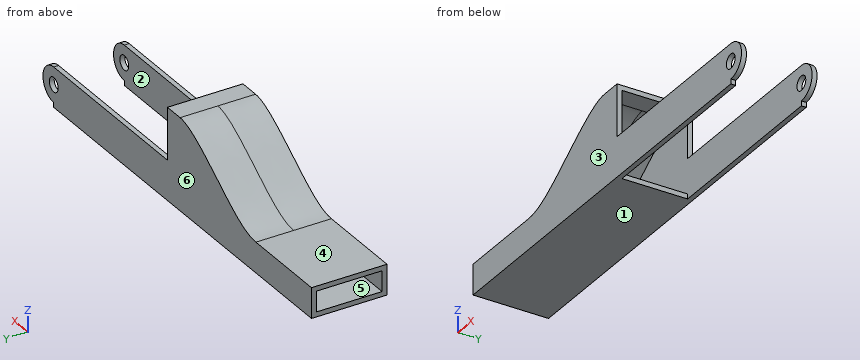
from build123d import *

# Parameters (mm, degrees)
F0_W     = 45
F0_H     = 8.5
F0_H_2   = 1.2
F0_W_2   = 22
F0_H_3   = 5
F1_DEPTH = 1.2
F2_DEPTH = 9.2
F3_D     = 3.5


# Not quite as in the source:
# - the dataset's text gives a spline's control points without its knots; the knots are read off the source's solid


with BuildPart() as f1:
    # F0 (on Front) → F1 (new body)
    with BuildSketch(Plane.XZ):
        with BuildLine():
            Line((47.5, -1.5), (47.5, -10))
            ThreePointArc((47.5, -10), (51.75, -5.75), (47.5, -1.5))
        make_face()
        with Locations((25, -5.75)):
            Rectangle(F0_W, F0_H)
        with Locations((25, -10.6)):
            Rectangle(F0_W, F0_H_2)
        with BuildLine():
            Line((-32.5, -10), (-2.5, -10))
            Line((-2.5, -10), (-2.5, 10))
            add(Edge.make_bspline(
                [(-32.5, -5), (-27.5803674012, -5), (-17.2100449751, 2.2275754238), (-6.0579581186, 10), (-2.5, 10)],
                knots=[0, 0, 0, 0, 0.5090778259, 1, 1, 1, 1], degree=3))
            Line((-32.5, -5), (-32.5, -10))
        make_face()
        Polygon((-2.5, -10), (2.5, -10), (2.5, -1.5), (2.5, 10), (-2.5, 10), align=None)
        with Locations((-43.5, -7.5)):
            Rectangle(F0_W_2, F0_H_3)
    extrude(amount=F1_DEPTH)

    # F0 (on Front) → F2 (join)
    with BuildSketch(Plane.XZ):
        with BuildLine():
            add(Edge.make_bspline(
                [(-32.5, -5), (-27.5803674012, -5), (-17.2100449751, 2.2275754238), (-6.0579581186, 10), (-2.5, 10)],
                knots=[0, 0, 0, 0, 0.5090778259, 1, 1, 1, 1], degree=3))
            Line((-2.5, 10), (2.5, 10))
            Line((2.5, 10), (2.5, 11.2))
            Line((2.5, 11.2), (-2.5, 11.2))
            add(Edge.make_bspline(
                [(-32.5, -3.8), (-31.4389363622, -3.8), (-29.2200835852, -3.4091842374), (-25.6037921172, -1.8183804645), (-21.7862624056, 0.5093473763), (-17.819156486, 3.2622809958), (-13.7265020427, 6.1236212623), (-10.3779360475, 8.2729183736), (-7.8194468713, 9.6607467479), (-5.973100675, 10.4877178879), (-4.2025331466, 11.0487112992), (-3.0621946213, 11.2), (-2.5, 11.2)],
                knots=[0, 0, 0, 0, 0.125, 0.25, 0.375, 0.5, 0.625, 0.75, 0.8125, 0.875, 0.9375, 1, 1, 1, 1], degree=3))
            Line((-32.5, -3.8), (-54.5, -3.8))
            Line((-54.5, -3.8), (-54.5, -5))
            Line((-54.5, -5), (-32.5, -5))
        make_face()
        Polygon((2.5, -11.2), (2.5, -10), (-2.5, -10), (-32.5, -10), (-54.5, -10), (-54.5, -11.2), (-32.8350449828, -11.2), (-2.8350449828, -11.2), align=None)
    extrude(amount=F2_DEPTH)

    # F3 (through all)
    with Locations(Plane(origin=(0, 0, 0), x_dir=(1, 0, 0), z_dir=(0, 1, 0))):
        with Locations((47.5, 5.75)):
            Hole(F3_D / 2)

    # F4: F1 across face


with BuildPart() as f1_1:
    add(f1.part)
    add(f1.part.mirror(Plane(origin=(-26, -9.2, -10.6), x_dir=(1, 0, 0), z_dir=(0, -1, 0))))


solid = f1_1.part
Here's how the part is built. I have some questions about the finished solid (model axes, mm). Face numbers are marked on the shaded views. A direction names the side the tool comes from. Round coordinates to 2 decimals unless told otherwise and drop trailing zeros. Write each loop counter-clockwise with the first axis right and the second up, starting at its lowest first coordinate (ties: lowest second). Pieces come first, ordered by that corner, then holes.
1. For the marked faces 1 and 2, which set-ups out of +Z, -Z, +X, -X, +Y, -Y let a thin tool reach every point of the face, with its end or its side?
2. If we mould it in two halves opening along Y, with no side actions, what happens to the marked faces 3, 4, 5 and 6? For each: released by +Y, released by -Y, zero draft, split by the parting line, or undercut.
3. Will these pins go through, and if not, where does the flat tip stop? pin 1 Ø5 at (x, y) = (-38, -6.5) entering from +Z; pin 2 Ø1 at (x, y) = (26, -0.5) entering from +Z; pin 3 Ø4 at (x, y) = (-11, -6.5) entering from +Z.
4. Suppose I cut it at A-A (x = 31.5). List the corners of the cut face in (y, z) for me, and give its area (3 significant figures).
5. I need wall thicknesses on L1, parallel to Y at x = 32, z = -3; L2, parallel to X at y = -0.35, z = -5.75; L3, parallel to X at y = -4.75, z = -10.5. Which ranges of each line are inside material? Lowest first, please.
Answer sheet:
1. face 1: -Z, +X, -X, +Y, -Y
1. face 2: +X
2. face 3: released by -Y
2. face 4: zero draft
2. face 5: undercut
2. face 6: released by +Y
3. pin 1: stops at z = -3.8
3. pin 2: stops at z = -1.5
3. pin 3: stops at z = 9.01
4. outline: (-18.4, -11.2) - (-17.2, -11.2) - (-17.2, -1.5) - (-18.4, -1.5) - close; (-1.2, -11.2) - (0, -11.2) - (0, -1.5) - (-1.2, -1.5) - close
4. area: 23.3 mm2
5. L1: y = -18.4 to -17.2, -1.2 to 0
5. L2: x = -54.5 to 45.75, 49.25 to 51.75
5. L3: x = -54.5 to 2.5
